```python
from build123d import *

# Parameters (mm, degrees)
F0_W     = 69
F0_H     = 33
F0_W_2   = 5
F0_H_2   = 5
F0_R     = 1.55
F1_DEPTH = 25
F3_W     = 50
F3_H     = 31
F4_DEPTH = 2
F6_W     = 15.3119070455
F6_H     = 28.5653881729
F7_DEPTH = 2
F8_W     = 5
F8_H     = 29.938359429
F8_R     = 1.55
F9_DEPTH = 2


with BuildPart() as f1:
    # F0 (on Top) → F1 (new body)
    with BuildSketch(Plane.XY):
        with Locations((32.5, -14.5)):
            Rectangle(F0_W, F0_H)
        Polygon((0, -5), (0, 0), (5, 0), (60, 0), (65, 0), (65, -5), (65, -24), (65, -29), (60, -29), (5, -29), (0, -29), (0, -24), align=None, mode=Mode.SUBTRACT)
        with Locations((2.5, -2.5)):
            Rectangle(F0_W_2, F0_H_2)
        with Locations((2.5, -2.5)):
            Circle(F0_R, mode=Mode.SUBTRACT)
        with Locations((62.5, -2.5)):
            Rectangle(F0_W_2, F0_H_2)
        with Locations((62.5, -2.5)):
            Circle(F0_R, mode=Mode.SUBTRACT)
        with Locations((62.5, -26.5)):
            Rectangle(F0_W_2, F0_H_2)
        with Locations((62.5, -26.5)):
            Circle(F0_R, mode=Mode.SUBTRACT)
        with Locations((2.5, -26.5)):
            Rectangle(F0_W_2, F0_H_2)
        with Locations((2.5, -26.5)):
            Circle(F0_R, mode=Mode.SUBTRACT)
    extrude(amount=F1_DEPTH)

    # F3 (on offset) → F4 (cut)
    with BuildSketch(Plane.XY.offset(16)):
        with Locations((32.9331636816, -14.5)):
            Rectangle(F3_W, F3_H)
    extrude(amount=F4_DEPTH, mode=Mode.SUBTRACT)

    # F6 (on offset) → F7 (cut)
    with BuildSketch(Plane.XY.offset(19)):
        with Locations((7.6559535228, -14.2826940864)):
            Rectangle(F6_W, F6_H)
    extrude(amount=F7_DEPTH, mode=Mode.SUBTRACT)

    # F8 (on Top) → F9 (join)
    with BuildSketch(Plane.XY):
        with Locations((20, -14.9691797145)):
            Rectangle(F8_W, F8_H)
        with Locations((20, -23)):
            Circle(F8_R, mode=Mode.SUBTRACT)
        with Locations((20, -6)):
            Circle(F8_R, mode=Mode.SUBTRACT)
        with Locations((45, -14.9691797145)):
            Rectangle(F8_W, F8_H)
        with Locations((45, -23)):
            Circle(F8_R, mode=Mode.SUBTRACT)
        with Locations((45, -6)):
            Circle(F8_R, mode=Mode.SUBTRACT)
    extrude(amount=F9_DEPTH)


solid = f1.part
```
CAD build for the part. Positions are in the model's coordinates, mm. A direction names the side the tool comes from. Coordinates: 2 decimals unless noted, no trailing zeros. Loops run counter-clockwise (first coordinate to the right, second up) from the corner with the lowest first, then second, coordinate; pieces in that order, holes last. Notation, with made-up numbers: (74, 68) - (112, 68) arc R25 ccw to (112, 90) - close; hole circle Ø2 at (29, 24.5). An arc over 180 degrees is marked (long way). Return JSON: item names as keys, results as strings.
1. Band-saw the part on B-B (y = -2.5). State how many separate pieces and enclosed holes the cut face has, and give its area (3 significant figures).
Result:
{"separate pieces": "7", "enclosed holes": "0", "area": "211 mm2"}
2. 3-axis set-ups, long thin cutter, end or side, ignore diameter. For faces 4 (the flat face through (17.5, -15, 1)), 5 (the flat face through (1, -1, 21)): which of +Z, -Z, +X, -X, +Y, -Y reach the whole face in a straight line?
Result:
{"face 4": "+Z, -Z", "face 5": "none"}
3. Probe L1, parallel to Y at x = 45, z = 0.8; L2, parallel to Y at x = 2.5, z = 22.15; L3, parallel to X at y = -17.5, z = 13.5. List the from-to ranges inside material, lowest first. Write a range as from..to.
Result:
{"L1": "y = -31..-24.55, -21.45..-7.55, -4.45..2", "L2": "y = -31..-28.05, -24.95..-24, -5..-4.05, -0.95..2", "L3": "x = -2..0, 65..67"}
4. Drop flat-ended pins along their axis: pin 1 (1.5 mm diameter, centred on x = 44.5, y = -10.5, fed in from +Z); pin 2 (1.9 mm diameter, centred on x = 2.5, y = -26.5, fed in from -Z). Give the stop position or say it passes through.
Result:
{"pin 1": "stops at z = 2", "pin 2": "passes through"}
5. Mould opens along Z. For faces 1 (the flat face through (22, -16, 0)), 2 (the flat face through (2, -24, 23)), 3 (the flat face through (2.5, -24.7, 19)) say: released by +Z, released by -Z, zero draft, split by the parting line, or undercut.
Result:
{"face 1": "released by -Z", "face 2": "zero draft", "face 3": "undercut"}
6. Band-saw the part on D-D (z = 22.25). Give the cut face in (x, y), and give its area (3 significant figures).
Result:
{"outline": "(-2, -31) - (67, -31) - (67, 2) - (-2, 2) - close; hole (0, -24) - (5, -24) - (5, -29) - (60, -29) - (60, -24) - (65, -24) - (65, -5) - (60, -5) - (60, 0) - (5, 0) - (5, -5) - (0, -5) - close; hole circle Ø3.1 at (2.5, -26.5); hole circle Ø3.1 at (2.5, -2.5); hole circle Ø3.1 at (62.5, -26.5); hole circle Ø3.1 at (62.5, -2.5)", "area": "462 mm2"}
7. Band-saw the part on A-A (x = 45). Give the cut face in (y, z), and give its area (3 significant figures).
Result:
{"outline": "(-31, 0) - (-24.55, 0) - (-24.55, 2) - (-29, 2) - (-29, 16) - (-30, 16) - (-30, 18) - (-29, 18) - (-29, 25) - (-31, 25) - close; (-21.45, 0) - (-7.55, 0) - (-7.55, 2) - (-21.45, 2) - close; (-4.45, 0) - (2, 0) - (2, 25) - (0, 25) - (0, 18) - (1, 18) - (1, 16) - (0, 16) - (0, 2) - (-4.45, 2) - close", "area": "142 mm2"}
